Design review of the part built by this model. Coordinates are the model's own, in mm. A direction names the side the tool comes from. Coordinates: 2 decimals unless noted, no trailing zeros. Loops run counter-clockwise (first coordinate to the right, second up) from the corner with the lowest first, then second, coordinate; pieces in that order, holes last. Notation, with made-up numbers: M -27.75,56 L 18.25,56 A20 ccw 18.25,72 Z; hole C 43.25,34.5 d1. An arc over 180 degrees is marked long. Put each result on its own line as item: value. Start each with the question number.
(1) Take a section at D-D, the plane x = -4. Give the boundary of the cut face in (y, z).
(2) For faces 1 (the flat face through (-55, 11, 8)), 2 (the flat face through (41, 3, 8)), 3 (the flat face through (-4, 4, 8)), list the 3-axis set-ups (+Z, -Z, +X, -X, +Y, -Y) from which the entire face can be reached by the end or side of a thin tool; tool diameter is ignored.
(3) For probe 1 along Z at (x, y) = (-25.69, -8); probe 2 along Y at (x, z) = (-52, 2.5); probe 3 along Y at (x, z) = (-10, 9.25), list the stretches that pass through material, from the lowest coordinate up. Write a range as [from, to].
(4) Take a section at B-B, the plane x = -25.69. Give the boundary of the cut face in (y, z), then the cut area to 3 significant figures.
(5) Take a section at A-A, the plane x = -51.5. Give the boundary of the cut face in (y, z), then the cut area to 3 significant figures.
(6) The part is to be moulded in two halves that separate along Z. For faces 4 (the cylindrical face through (-28.55, 8.52, 8.9)), 5 (the cylindrical face through (78.961, 0.042, 13.594)), 6 (the cylindrical face through (-92.35, 8.48, 2.28)), 7 (the cylindrical face through (-83.76, 8.52, 8.13)), say which applies: +Z half, -Z half, draft (parallel to the pull), parting line (faces both ways), or undercut.
(7) Clearance check with flat-ended pins moving along their axes: pin 1 (3.5 mm diameter, centred on x = -86.76, z = 8, fed in from +Y); pin 2 (9.5 mm diameter, centred on x = -25.69, z = 8, fed in from -Y); pin 3 (7 mm diameter, centred on x = -89, z = 9, fed in from -Y); pin 4 (2 mm diameter, centred on x = 62, z = 5, fed in from +Y). State where each tip first meets the part, or that it passes through.
```python
from build123d import *

# Parameters (mm, degrees)
F1_DEPTH = 16
F3_W     = 3
F3_H     = 16
F5_DEPTH = 8
F4_W     = 6
F4_H     = 16
F6_DEPTH = 8
F7_D     = 6
F8_R     = 7.99999


# Not quite as in the source:
# - a fillet or chamfer is up to 0.001 mm smaller than in the source, because OpenCascade refuses the exact size


with BuildPart() as f1:
    # F0 (on Top) → F1 (new body)
    with BuildSketch(Plane.XY):
        Polygon((-80.7573593129, 10), (-86.7573593129, 10), (-86.7573593129, 7), (-80.0491553804, 7), (-72.0491553804, 11), (-38.4655632454, 11), (-30.4655632454, 7), (-7, 7), (0, 0), (-7, -7), (-30.4655632454, -7), (-38.4655632454, -11), (-72.0491553804, -11), (-80.0491553804, -7), (-86.7573593129, -7), (-86.7573593129, -10), (-80.7573593129, -10), (-72.7573593129, -14), (-37.7573593129, -14), (-29.7573593129, -10), (-5.7573593129, -10), (1.2426406871, -3), (73.2426406871, -3), (73.2426406871, 3), (1.2426406871, 3), (-5.7573593129, 10), (-29.7573593129, 10), (-37.7573593129, 14), (-72.7573593129, 14), align=None)
    extrude(amount=F1_DEPTH)

    # F3 (on face) → F5 (join)
    with BuildSketch(Plane(origin=(-86.7573593129, 0, 0), x_dir=(0, -1, 0), z_dir=(-1, 0, 0))):
        with Locations((-8.5, 8)):
            Rectangle(F3_W, F3_H)
        with Locations((8.5, 8)):
            Rectangle(F3_W, F3_H)
    extrude(amount=F5_DEPTH)

    # F4 (on face) → F6 (join)
    with BuildSketch(Plane.YZ.offset(73.2426406871)):
        with Locations((0, 8)):
            Rectangle(F4_W, F4_H)
    extrude(amount=F6_DEPTH)

    # F7 (through all)
    with Locations(Plane.XZ.offset(10)):
        with Locations((-86.7573593129, 8), (-25.6900005043, 8)):
            Hole(F7_D / 2)

    # F8 (radius 8 in the source; OpenCascade refuses exactly that, so slightly less here)
    f8_edges = [f1.edges().sort_by_distance(p)[0] for p in [
        (-94.757359, -8.5, 16),
        (-94.757359, -8.5, 0),
        (-94.757359, 8.5, 0),
        (-94.757359, 8.5, 16),
        (81.242641, 0, 16),
        (81.242641, 0, 0),
    ]]
    fillet(f8_edges, radius=F8_R)


solid = f1.part
```
Computed values:
1. outline: M -8.24,0 L -4,0 L -4,16 L -8.24,16 Z; M 4,0 L 8.24,0 L 8.24,16 L 4,16 Z
2. face 1: +Z, -Z
2. face 2: +Z, -Z, +X, +Y
2. face 3: +Z, -Z, -X
3. probe 1: z = [0, 5], [11, 16]
3. probe 2: y = [-14, -11], [11, 14]
3. probe 3: y = [-10, -7], [7, 10]
4. outline: M -10,0 L -7,0 L -7,5 L -10,5 Z; M -10,11 L -7,11 L -7,16 L -10,16 Z; M 7,0 L 10,0 L 10,5 L 7,5 Z; M 7,11 L 10,11 L 10,16 L 7,16 Z
4. area: 60.0 mm^2
5. outline: M -14,0 L -11,0 L -11,16 L -14,16 Z; M 11,0 L 14,0 L 14,16 L 11,16 Z
5. area: 96.0 mm^2
6. face 4: undercut
6. face 5: +Z half
6. face 6: -Z half
6. face 7: undercut
7. pin 1: passes through
7. pin 2: stops at y = -10.34
7. pin 3: stops at y = -10
7. pin 4: stops at y = 3
